Check sheet for the modelled part. Datum: model origin and axes. Units: mm. Face numbers are marked on the shaded views. Give positions to 0.01 mm unless a question says otherwise; leave off trailing zeros. Write each loop counter-clockwise with the first axis right and the second up, starting at its lowest first coordinate (ties: lowest second). Pieces come first, ordered by that corner, then holes. Notation, with made-up numbers: M 84.25,86.5 L 114.25,86.5 A26 cw 114.25,114.5 Z; hole C 50,47 d9. An arc over 180 degrees is marked long. Write each question's results on one line, items separated by ' | '. Start each with the question number.
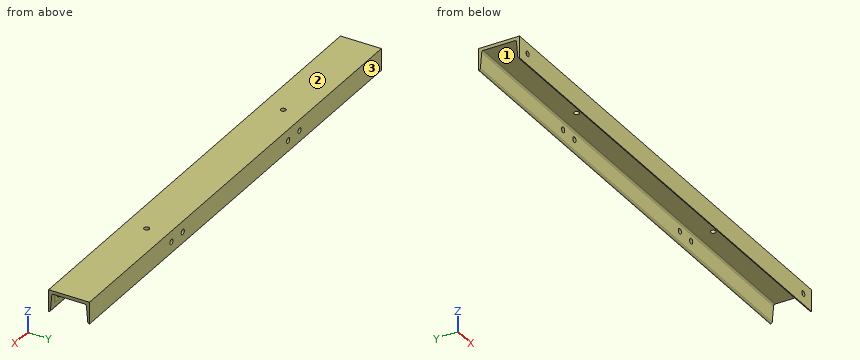
from build123d import *

# Parameters (mm, degrees)
STRUCTURAL_MEMBER1_DEPTH = 900
SKETCH12_R               = 4.7625
CUT_EXTRUDE1_DEPTH       = 454.327971782
CUT_EXTRUDE2_DEPTH       = 40
SKETCH16_R               = 4.7625
CUT_EXTRUDE3_DEPTH       = 454.327971881
SKETCH17_R               = 4.7625
CUT_EXTRUDE4_DEPTH       = 454.327971881


with BuildPart() as part:
    # Sketch112 → Structural Member1 (new body)
    with BuildSketch(Plane(origin=(-450, 0, 0), x_dir=(0, 0, 1), z_dir=(1, 0, 0))):
        with BuildLine():
            Line((0, 37.5), (0, -37.5))
            Line((0, -37.5), (-40, -37.5))
            Line((-40, -37.5), (-40, -37.246949676))
            ThreePointArc((-40, -37.246949676), (-39.212582687, -35.220998578), (-37.263681431, -34.258560126))
            Line((-37.263681431, -34.258560126), (-8.736318569, -31.741439874))
            ThreePointArc((-8.736318569, -31.741439874), (-6.787417313, -30.779001422), (-6, -28.753050324))
            Line((-6, -28.753050324), (-6, 28.753050324))
            ThreePointArc((-6, 28.753050324), (-6.787417313, 30.779001422), (-8.736318569, 31.741439874))
            Line((-8.736318569, 31.741439874), (-37.263681431, 34.258560126))
            ThreePointArc((-37.263681431, 34.258560126), (-39.212582687, 35.220998578), (-40, 37.246949676))
            Line((-40, 37.246949676), (-40, 37.5))
            Line((-40, 37.5), (0, 37.5))
        make_face()
    extrude(amount=STRUCTURAL_MEMBER1_DEPTH)

    # Sketch12 → Cut-Extrude1 (cut, through all)
    with BuildSketch(Plane(origin=(0, 0, 0), x_dir=(1, 0, 0), z_dir=(0, 1, 0))):
        with Locations(Location((-425, 20, 0), (0, 0, 270))):
            Circle(SKETCH12_R)
        with Locations(Location((425, 20, 0), (0, 0, 270))):
            Circle(SKETCH12_R)
    extrude(amount=-CUT_EXTRUDE1_DEPTH, mode=Mode.SUBTRACT)

    # Sketch15 → Cut-Extrude2 (cut)
    with BuildSketch(Plane(origin=(0, 0, -6), x_dir=(-1, 0, 0), z_dir=(0, 0, -1))):
        with BuildLine():
            Line((-412.5, -33.5), (-437.5, -33.5))
            ThreePointArc((-437.5, -33.5), (-442.5, -28.5), (-437.5, -23.5))
            Line((-437.5, -23.5), (-412.5, -23.5))
            ThreePointArc((-412.5, -23.5), (-407.5, -28.5), (-412.5, -33.5))
        make_face()
        with BuildLine():
            Line((412.5, -33.5), (437.5, -33.5))
            ThreePointArc((437.5, -33.5), (442.5, -28.5), (437.5, -23.5))
            Line((437.5, -23.5), (412.5, -23.5))
            ThreePointArc((412.5, -23.5), (407.5, -28.5), (412.5, -33.5))
        make_face()
    extrude(amount=CUT_EXTRUDE2_DEPTH, mode=Mode.SUBTRACT)

    # Sketch16 → Cut-Extrude3 (cut, through all)
    with BuildSketch(Plane(origin=(0, 0, 0), x_dir=(1, 0, 0), z_dir=(0, 1, 0))):
        with Locations(Location((-197.5, 20, 0), (0, 0, 270))):
            Circle(SKETCH16_R)
        with Locations(Location((-162.5, 20, 0), (0, 0, 270))):
            Circle(SKETCH16_R)
        with Locations(Location((162.5, 20, 0), (0, 0, 90))):
            Circle(SKETCH16_R)
        with Locations(Location((197.5, 20, 0), (0, 0, 90))):
            Circle(SKETCH16_R)
    extrude(amount=CUT_EXTRUDE3_DEPTH, mode=Mode.SUBTRACT)

    # Sketch17 → Cut-Extrude4 (cut, through all)
    with BuildSketch(Plane.XY):
        with Locations((-210.6, 0)):
            Circle(SKETCH17_R)
        with Locations((210.6, 0)):
            Circle(SKETCH17_R)
    extrude(amount=-CUT_EXTRUDE4_DEPTH, mode=Mode.SUBTRACT)


solid = part.part
Q1. Release check for a two-part mould opening along Y. For the marked faces 1, 2 and 3 record: pulls with the +Y half, pulls with the -Y half, needs draft (parallel to the pull), parting line crosses it, or undercut.
Q2. Depth check by flat-ended pin: pin 1 Ø1 at (x, y) = (65.5, 18.5) entering from -Z; pin 2 Ø5.5 at (x, z) = (-425, -20) entering from -Y; pin 3 Ø8 at (x, y) = (-82, -26.5) entering from -Z. Enter the tip coordinate at first touch or a pass-through.
Q3. Section check B-B on y = 18. Record the boundary of the cut face in (x, z).
Q4. Section check A-A on x = -94.5. Record the boundary of the cut face in (y, z), plus the area to 3 significant figures.
Q5. Scan lines: L1, parallel to X at y = 34.75, z = -20; L2, parallel to X at y = -32.5, z = -13; L3, parallel to Z at x = 250, y = 10. Record each from-to range of solid material in increasing order.
Check result:
1) face 1: undercut | face 2: needs draft | face 3: pulls with the +Y half
2) pin 1: z = -6 | pin 2: y = 32.49 | pin 3: z = -6.56
3) outline: M -450,-6 L 450,-6 L 450,0 L -450,0 Z
4) outline: M -37.5,-40 L -37.25,-40 A3 ccw -34.26,-37.26 L -31.74,-8.74 A3 cw -28.75,-6 L 28.75,-6 A3 cw 31.74,-8.74 L 34.26,-37.26 A3 ccw 37.25,-40 L 37.5,-40 L 37.5,0 L -37.5,0 Z | area: 756 mm^2
5) L1: -450 to -202.26, -192.74 to -167.26, -157.74 to 157.74, 167.26 to 192.74, 202.26 to 450 | L2: -450 to -440.5, -409.5 to 409.5, 440.5 to 450 | L3: -6 to 0
